Geometry: final body of the model. Coordinates: model frame, mm. Face numbers are marked on the shaded views. A direction names the side the tool comes from. Give positions to 0.01 mm unless a question says otherwise; leave off trailing zeros. Loops run counter-clockwise (first coordinate to the right, second up) from the corner with the lowest first, then second, coordinate; pieces in that order, holes last.
Solid Edge part; units mm, degrees
sketch "Sketch1" plane through (0, 0, 0) normal (0, -1, 0) x (1, 0, 0)
  line L0 (14, -13.5) -> (-14, -13.5)
  line L1 (-14, -13.5) -> (-14, 13.5)
  line L2 (-14, 13.5) -> (14, 13.5)
  line L3 (14, 13.5) -> (14, -13.5)
  dimension "D1" = 14
  dimension "D2" = 14
extrude "Protrusion1" add sketch "Sketch1" along normal mid plane 10
sketch "Sketch2" plane through (0, -2.5, 0) normal (0, -1, 0) x (1, 0, 0)
  circle A0 centre (0, 13.5) radius 10.5
extrude "Extrusionsausschnitt_1" cut sketch "Sketch2" against normal blind 5
fillet "Verrundung_1" radius 1 8 edges at (-14, -5, 0) (14, -5, 0) (-14, 5, 0) (14, 5, 0) (0, -5, -13.5) (-14, 0, -13.5) (0, 5, -13.5) (14, 0, -13.5)
sketch "Sketch3" plane through (0, -5, 0.5) normal (0, -1, 0) x (1, 0, 0)
  circle A0 centre (0, 13) radius 7.5
extrude "Extrusionsausschnitt_2" cut sketch "Sketch3" against normal blind 19.0261
hole "Bohrung_1" at (-7, 0, -13.5) direction (0, 0, 1) diameter 2.459 depth 8
hole "Hole1" at (7, 0, -13.5) direction (0, 0, 1) diameter 2.459 depth 8
properties part number "037" material "PLA"
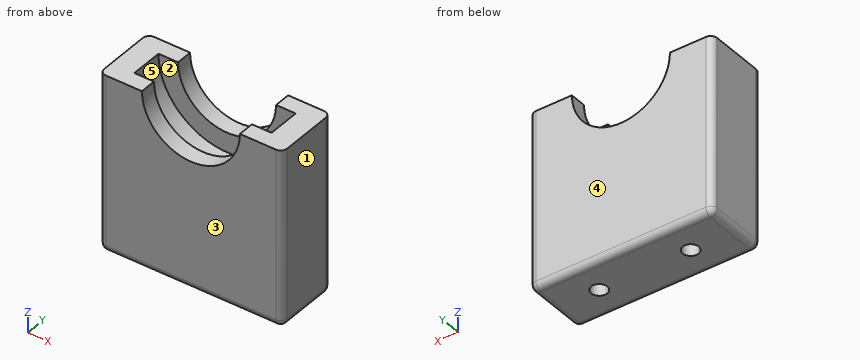
Item 1: Pin query (flat end, axial travel): pin 1 (2 mm diameter, centred on x = 7.5, y = 0, fed in from -Z); pin 2 (3 mm diameter, centred on x = 7, y = 0, fed in from +Z). Return the tip coordinate at first contact, or that it passes through.
Values follow:
pin 1: stops at z = -13.5
pin 2: stops at z = 7.34
Item 2: Section query B-B on y = 3.5. Return loops of the section in (x, z).
Values follow:
outline: (-14, -12.5) arc R1 ccw to (-13, -13.5) - (13, -13.5) arc R1 ccw to (14, -12.5) - (14, 13.5) - (7.5, 13.5) arc R7.5 cw to (-7.5, 13.5) - (-14, 13.5) - close
Item 3: Ray query, probe 1 along X at (y, z) = (0, -9); probe 2 along Y at (x, z) = (-7, -11.25); probe 3 along Y at (x, z) = (-6.5, 7). Return the intervals inside material, ascending.
Values follow:
probe 1: x = -14 to -8.23, -5.77 to 5.77, 8.23 to 14
probe 2: y = -5 to -1.23, 1.23 to 5
probe 3: y = -5 to -2.5, 2.5 to 5
Item 4: Draft query along X for the marked faces 1, 2 and 3. Return one class per face: +X half, -X half, draft (parallel to the pull), parting line (faces both ways), or undercut.
Values follow:
face 1: +X half
face 2: undercut
face 3: draft
Item 5: Section query C-C on z = 10.25. Return loops of the section in (x, y), plus the area to 3 significant figures.
Values follow:
outline: (-14, -4) arc R1 ccw to (-13, -5) - (-6.76, -5) - (-6.76, -2.5) - (-9.98, -2.5) - (-9.98, 2.5) - (-6.76, 2.5) - (-6.76, 5) - (-13, 5) arc R1 ccw to (-14, 4) - close; (6.76, -5) - (13, -5) arc R1 ccw to (14, -4) - (14, 4) arc R1 ccw to (13, 5) - (6.76, 5) - (6.76, 2.5) - (9.98, 2.5) - (9.98, -2.5) - (6.76, -2.5) - close
area: 112 mm2
Item 6: Set-up query: the marked faces 4 and 5. Return all of +Z, -Z, +X, -X, +Y, -Y with unobstructed straight access to the full face (end or side cutting, diameter ignored); none if empty.
Values follow:
face 4: +Z, -Z, +X, -X, +Y
face 5: +Z
Item 7: Section query A-A on z = -9.25. Return loops of the section in (x, y).
Values follow:
outline: (-14, -4) arc R1 ccw to (-13, -5) - (13, -5) arc R1 ccw to (14, -4) - (14, 4) arc R1 ccw to (13, 5) - (-13, 5) arc R1 ccw to (-14, 4) - close; hole circle Ø2.46 at (-7, 0); hole circle Ø2.46 at (7, 0)
Item 8: Section query D-D on x = 0. Return loops of the section in (y, z).
Values follow:
outline: (-5, -12.5) arc R1 ccw to (-4, -13.5) - (4, -13.5) arc R1 ccw to (5, -12.5) - (5, 6) - (2.5, 6) - (2.5, 3) - (-2.5, 3) - (-2.5, 6) - (-5, 6) - close
